The listing builds one solid part. Answer for the finished solid, in the listing's coordinates (mm). A direction names the side the tool comes from. Round coordinates to 2 decimals unless told otherwise and drop trailing zeros. Loops run counter-clockwise (first coordinate to the right, second up) from the corner with the lowest first, then second, coordinate; pieces in that order, holes last. Notation, with made-up numbers: (-9.5, -10) - (49.5, -10) arc R26 ccw to (49.5, 7) - close; hole circle Ø9 at (50, 14.5). An arc over 180 degrees is marked (long way). One line per item, written item: value.
```python
from build123d import *

# Parameters (mm, degrees)
EXTRUDE_1_DEPTH = 1010
FILLET_1_R      = 2
FILLET_2_R      = 0.5
FILLET_3_R      = 0.5
FILLET_4_R      = 3


with BuildPart() as part:
    # 草图1 → 凸台-拉伸1 (new body)
    with BuildSketch(Plane.XY):
        Polygon((-52, 0), (-27, 0), (-27, 2), (-50, 2), (-50, 18), (78.43916289, 18), (78.43916289, 2), (57.650269721, 2), (57.650269721, 0), (80.43916289, 0), (80.43916289, 20), (58, 20), (58, 28), (52, 28), (52, 34), (58, 34), (58, 42), (18, 42), (18, 34), (24, 34), (24, 28), (18, 28), (18, 20), (-52, 20), align=None)
    extrude(amount=-EXTRUDE_1_DEPTH)

    # 圆角1
    fillet_1_edges = [part.edges().sort_by_distance(p)[0] for p in [
        (80.43916289, 20, -505),
        (80.43916289, 0, -505),
        (-52, 0, -505),
        (-52, 20, -505),
    ]]
    fillet(fillet_1_edges, radius=FILLET_1_R)

    # 圆角2
    fillet_2_edges = [part.edges().sort_by_distance(p)[0] for p in [
        (57.650269721, 0, -505),
        (57.650269721, 2, -505),
        (-27, 2, -505),
        (-27, 0, -505),
    ]]
    fillet(fillet_2_edges, radius=FILLET_2_R)

    # 圆角3
    fillet_3_edges = [part.edges().sort_by_distance(p)[0] for p in [
        (57.650269721, 1, 0),
        (57.650269721, 1, -1010),
        (-38.75, 0, 0),
        (-27, 1, 0),
        (-38.75, 2, 0),
        (-27.146446609, 1.853553391, 0),
        (-27.146446609, 0.146446609, 0),
        (57.79671633, 1.853553391, 0),
        (57.79671633, 0.146446609, 0),
        (-38.75, 2, -1010),
        (-27, 1, -1010),
        (-38.75, 0, -1010),
        (-27.146446609, 1.853553391, -1010),
        (-27.146446609, 0.146446609, -1010),
        (57.79671633, 1.853553391, -1010),
        (57.79671633, 0.146446609, -1010),
        (68.294716305, 2, -1010),
        (68.219581445, 20, -1010),
        (68.294716305, 2, 0),
        (68.219581445, 20, 0),
        (68.294716305, 0, 0),
        (68.294716305, 0, -1010),
        (-16, 20, 0),
        (-52, 10, 0),
        (80.43916289, 10, 0),
        (-51.414213562, 19.414213562, 0),
        (-51.414213562, 0.585786438, 0),
        (79.853376452, 19.414213562, 0),
        (79.853376452, 0.585786438, 0),
        (80.43916289, 10, -1010),
        (-52, 10, -1010),
        (-16, 20, -1010),
        (-51.414213562, 19.414213562, -1010),
        (-51.414213562, 0.585786438, -1010),
        (79.853376452, 19.414213562, -1010),
        (79.853376452, 0.585786438, -1010),
    ]]
    fillet(fillet_3_edges, radius=FILLET_3_R)

    # 圆角4
    fillet_4_edges = [part.edges().sort_by_distance(p)[0] for p in [
        (58, 34, -505),
        (58, 28, -505),
        (18, 28, -505),
        (18, 34, -505),
    ]]
    fillet(fillet_4_edges, radius=FILLET_4_R)

    # 放样1: read off the stored shape, not the designer's step
    # 放样1: loft between two sections, ruled curve by curve
    loft_1_from = [
        Edge.make_bspline([(70.846246082, -10, -13.004005958), (81.838234165, -10, -17.818172342), (77.024067781, -10, -28.810160426), (66.032079698, -10, -23.995994042), (55.040091614, -10, -19.181827658), (59.854257998, -10, -8.189839574), (70.846246082, -10, -13.004005958)], [0, 0, 0, 0, 0.5, 0.5, 0.5, 1, 1, 1, 1], 3, [1, 0.333333333, 0.333333333, 1, 0.333333333, 0.333333333, 1]),
    ]
    loft_1_to = [
        Edge.make_bspline([(68.192900935, 0, -10.503791208), (84.185318519, 0, -10.011267297), (84.67784243, 0, -26.003684881), (68.685424845, 0, -26.496208792), (52.693007261, 0, -26.988732703), (52.20048335, 0, -10.996315119), (68.192900935, 0, -10.503791208)], [0, 0, 0, 0, 0.5, 0.5, 0.5, 1, 1, 1, 1], 3, [1, 0.333333333, 0.333333333, 1, 0.333333333, 0.333333333, 1]),
    ]
    loft_1 = Solid(Shell([*[Face.make_surface_from_curves(loft_1_from[k], loft_1_to[k]) for k in range(1)], Face(Wire(loft_1_from)), Face(Wire(loft_1_to))]))
    add(loft_1)

    # 阵列(线性)1: read off the stored shape, not the designer's step
    # 阵列(线性)1: loft between two sections, ruled curve by curve
    pattern_linear_1_from = [
        Edge.make_bspline([(70.846246082, -10, -987.004005958), (81.838234165, -10, -991.818172342), (77.024067781, -10, -1002.810160426), (66.032079698, -10, -997.995994042), (55.040091614, -10, -993.181827658), (59.854257998, -10, -982.189839574), (70.846246082, -10, -987.004005958)], [0, 0, 0, 0, 0.5, 0.5, 0.5, 1, 1, 1, 1], 3, [1, 0.333333333, 0.333333333, 1, 0.333333333, 0.333333333, 1]),
    ]
    pattern_linear_1_to = [
        Edge.make_bspline([(68.192900935, 0, -984.503791208), (84.185318519, 0, -984.011267297), (84.67784243, 0, -1000.003684881), (68.685424845, 0, -1000.496208792), (52.693007261, 0, -1000.988732703), (52.20048335, 0, -984.996315119), (68.192900935, 0, -984.503791208)], [0, 0, 0, 0, 0.5, 0.5, 0.5, 1, 1, 1, 1], 3, [1, 0.333333333, 0.333333333, 1, 0.333333333, 0.333333333, 1]),
    ]
    pattern_linear_1 = Solid(Shell([*[Face.make_surface_from_curves(pattern_linear_1_from[k], pattern_linear_1_to[k]) for k in range(1)], Face(Wire(pattern_linear_1_from)), Face(Wire(pattern_linear_1_to))]))
    add(pattern_linear_1)

    # Pattern Linear 1 2: loft between two sections, ruled curve by curve
    pattern_linear_1_2_from = [
        Edge.make_bspline([(-35.153753918, -10, -13.004005958), (-24.161765835, -10, -17.818172342), (-28.975932219, -10, -28.810160426), (-39.967920302, -10, -23.995994042), (-50.959908386, -10, -19.181827658), (-46.145742002, -10, -8.189839574), (-35.153753918, -10, -13.004005958)], [0, 0, 0, 0, 0.5, 0.5, 0.5, 1, 1, 1, 1], 3, [1, 0.333333333, 0.333333333, 1, 0.333333333, 0.333333333, 1]),
    ]
    pattern_linear_1_2_to = [
        Edge.make_bspline([(-37.807099065, 0, -10.503791208), (-21.814681481, 0, -10.011267297), (-21.32215757, 0, -26.003684881), (-37.314575155, 0, -26.496208792), (-53.306992739, 0, -26.988732703), (-53.79951665, 0, -10.996315119), (-37.807099065, 0, -10.503791208)], [0, 0, 0, 0, 0.5, 0.5, 0.5, 1, 1, 1, 1], 3, [1, 0.333333333, 0.333333333, 1, 0.333333333, 0.333333333, 1]),
    ]
    pattern_linear_1_2 = Solid(Shell([*[Face.make_surface_from_curves(pattern_linear_1_2_from[k], pattern_linear_1_2_to[k]) for k in range(1)], Face(Wire(pattern_linear_1_2_from)), Face(Wire(pattern_linear_1_2_to))]))
    add(pattern_linear_1_2)

    # Pattern Linear 1 3: loft between two sections, ruled curve by curve
    pattern_linear_1_3_from = [
        Edge.make_bspline([(-35.153753918, -10, -987.004005958), (-24.161765835, -10, -991.818172342), (-28.975932219, -10, -1002.810160426), (-39.967920302, -10, -997.995994042), (-50.959908386, -10, -993.181827658), (-46.145742002, -10, -982.189839574), (-35.153753918, -10, -987.004005958)], [0, 0, 0, 0, 0.5, 0.5, 0.5, 1, 1, 1, 1], 3, [1, 0.333333333, 0.333333333, 1, 0.333333333, 0.333333333, 1]),
    ]
    pattern_linear_1_3_to = [
        Edge.make_bspline([(-37.807099065, 0, -984.503791208), (-21.814681481, 0, -984.011267297), (-21.32215757, 0, -1000.003684881), (-37.314575155, 0, -1000.496208792), (-53.306992739, 0, -1000.988732703), (-53.79951665, 0, -984.996315119), (-37.807099065, 0, -984.503791208)], [0, 0, 0, 0, 0.5, 0.5, 0.5, 1, 1, 1, 1], 3, [1, 0.333333333, 0.333333333, 1, 0.333333333, 0.333333333, 1]),
    ]
    pattern_linear_1_3 = Solid(Shell([*[Face.make_surface_from_curves(pattern_linear_1_3_from[k], pattern_linear_1_3_to[k]) for k in range(1)], Face(Wire(pattern_linear_1_3_from)), Face(Wire(pattern_linear_1_3_to))]))
    add(pattern_linear_1_3)


solid = part.part
```
1) For faces 4 (the flat face through (78.439, 10, -498)), 5 (the flat face through (-16, 20, -498)), 6 (the flat face through (68, 20, -498)), determine the directions among +Z, -Z, +X, -X, +Y, -Y from which every point of the face is accessible in a straight line to the end or side of a thin tool.
Final values:
face 4: +Z, -Z
face 5: +Z, -Z, -X, +Y
face 6: +Z, -Z, +X, +Y
2) Each of these flat-tipped pins is pushed along its axis until it touches: pin 1 Ø3 at (y, z) = (22, -606.5) entering from -X; pin 2 Ø5 at (x, z) = (13.5, -436.5) entering from +Y; pin 3 Ø1.5 at (y, z) = (-0.5, -312) entering from +X. Where does it stop, or does it pass through?
Final values:
pin 1: x = 18
pin 2: y = 20
pin 3: x = 79.41
3) For a pull along Z with two mould halves and no side action, classify faces 1 (the flat face through (13, 18, -498)), 2 (the flat face through (33, 27, 0)), 3 (the flat face through (68, 0, -498)) as released by +Z, released by -Z, zero draft, split by the parting line, or undercut.
Final values:
face 1: zero draft
face 2: released by +Z
face 3: undercut
4) A cutting plane is placed at B-B on x = 40.5. Give the vertices of the cut face in (y, z).
Final values:
outline: (18, -1010) - (42, -1010) - (42, 0) - (18, 0) - close
5) A cutting plane is placed at A-A on x = -10. Give the vertices of the cut face in (y, z), and give its area (3 significant figures).
Final values:
outline: (18, -1010) - (19.5, -1010) arc R0.5 ccw to (20, -1009.5) - (20, -0.5) arc R0.5 ccw to (19.5, 0) - (18, 0) - close
area: 2,020 mm2
6) Consider L1, parallel to Y at x = -33, z = -388.5; L2, parallel to X at y = 16.5, z = -860; L3, parallel to Y at x = 11.5, z = -919. Determine where each line is inside the solid, lowest interval first.
Final values:
L1: 0 to 2, 18 to 20
L2: -52 to -50, 78.44 to 80.44
L3: 18 to 20
